```python
from build123d import *

# Parameters (mm, degrees)
F1_DEPTH = 3.175
F2_SIZE  = 0.254


with BuildPart() as f1:
    # F0 (on Front) → F1 (new body)
    with BuildSketch(Plane.XZ):
        with BuildLine():
            ThreePointArc((-9.178167, -7.9375), (-9.925332, -8.430318), (-9.766452, -9.31116))
            ThreePointArc((-9.766452, -9.31116), (13.49375, 0), (-9.766452, 9.31116))
            ThreePointArc((-9.766452, 9.31116), (-9.925332, 8.430318), (-9.178167, 7.9375))
            Line((-9.178167, 7.9375), (-5.504758, 7.9375))
            ThreePointArc((-5.504758, 7.9375), (-5.279535, 7.969327), (-5.071951, 8.062316))
            ThreePointArc((-5.071951, 8.062316), (9.525, 0), (-5.071951, -8.062316))
            ThreePointArc((-5.071951, -8.062316), (-5.279535, -7.969327), (-5.504758, -7.9375))
            Line((-5.504758, -7.9375), (-9.178167, -7.9375))
        make_face()
    extrude(amount=-F1_DEPTH)

    # F2
    f2_edges = [f1.edges().sort_by_distance(p)[0] for p in [
        (13.49375, 0, 0),
        (13.49375, 3.175, 0),
    ]]
    chamfer(f2_edges, length=F2_SIZE)


solid = f1.part
```
Input: part model. Units: mm. Frame: model coordinates. A direction names the side the tool comes from. Coordinates: 2 decimals unless noted, no trailing zeros. Write each loop counter-clockwise with the first axis right and the second up, starting at its lowest first coordinate (ties: lowest second). Pieces come first, ordered by that corner, then holes.
1) Material intervals for line 1 along Z through (x, y) = (0, 2.3) (3 decimals); line 2 along X through (y, z) = (1.05, 0) (3 decimals); line 3 along Z through (x, y) = (-3.5, 1.8), sorted ascending.
2) Mould query, pull axis Z, two halves, no side actions, for faces 1 (the cylindrical face through (13.486, 1.569, -0.45)), 2 (the flat face through (9.4, 3.175, -3.9)), 3 (the cylindrical face through (-9.93, 1.57, 8.44)), 4 (the cylindrical face through (9.52, 1.57, 0.28)). Classes: pulls with the +Z half, pulls with the -Z half, needs draft (parallel to the pull), parting line crosses it, or undercut.
3) Section B-B on z = 0. Output: boundary loops of the cut face in (x, y) (3 decimals), and give its area (3 significant figures).
4) Pin query (flat end, axial travel): pin 1 Ø1.3 at (x, y) = (-6.5, 2) entering from -Z; pin 2 Ø1 at (x, y) = (-7.5, 2) entering from +Z; pin 3 Ø1.3 at (x, y) = (-8, 2) entering from +Z. Return the tip coordinate at first contact, or that it passes through.
5) Section A-A on x = 0. Output: boundary loops of the cut face in (y, z) (3 decimals), and give its area (3 significant figures).
6) Set-up query: faces 5 (the flat face through (9.4, 0, -3.9)), 6 (the flat face through (-7, 2, -7.938)). Return all of +Z, -Z, +X, -X, +Y, -Y with unobstructed straight access to the full face (end or side cutting, diameter ignored); none if empty.
Check result:
1. line 1: z = -13.494 to -9.525, 9.525 to 13.494
1. line 2: x = 9.525 to 13.494
1. line 3: z = -13.03 to -8.86, 8.86 to 13.03
2. face 1: parting line crosses it
2. face 2: needs draft
2. face 3: undercut
2. face 4: undercut
3. outline: (9.525, 0.254) - (9.779, 0) - (13.24, 0) - (13.494, 0.254) - (13.494, 2.921) - (13.24, 3.175) - (9.779, 3.175) - (9.525, 2.921) - close
3. area: 12.5 mm2
4. pin 1: stops at z = -12.16
4. pin 2: stops at z = 11.54
4. pin 3: stops at z = 11.32
5. outline: (0, -13.24) - (0.254, -13.494) - (2.921, -13.494) - (3.175, -13.24) - (3.175, -9.779) - (2.921, -9.525) - (0.254, -9.525) - (0, -9.779) - close; (0, 9.779) - (0.254, 9.525) - (2.921, 9.525) - (3.175, 9.779) - (3.175, 13.24) - (2.921, 13.494) - (0.254, 13.494) - (0, 13.24) - close
5. area: 24.9 mm2
6. face 5: +Z, -Z, +X, -X, -Y
6. face 6: -X, +Y, -Y
